from build123d import *

# Parameters (mm, degrees)
SKETCH1_R                  = 75.438
BOSS_EXTRUDE1_DEPTH        = 3.175
SKETCH2_R                  = 3.175
CUT_EXTRUDE1_DEPTH         = 107.732676875
SKETCH3_R                  = 7
SKETCH3_R_2                = 2
CUT_EXTRUDE2_DEPTH         = 107.732676875
F_1_2_0_5_DIAMETER_HOLE1_D = 12.7


with BuildPart() as part:
    # Sketch1 → Boss-Extrude1 (new body)
    with BuildSketch(Plane(origin=(0, 0, 0), x_dir=(1, 0, 0), z_dir=(0, 1, 0))):
        with Locations(Location((0, 0, 0), (0, 0, 270))):
            Circle(SKETCH1_R)
    extrude(amount=BOSS_EXTRUDE1_DEPTH)

    # Sketch2 → Cut-Extrude1 (cut, through all)
    with BuildSketch(Plane(origin=(0, 3.175, 0), x_dir=(1, 0, 0), z_dir=(0, 1, 0))):
        with Locations(Location((50.8, 0, 0), (0, 0, 270))):
            Circle(SKETCH2_R)
        with Locations(Location((-50.8, 0, 0), (0, 0, 90))):
            Circle(SKETCH2_R)
    extrude(amount=-CUT_EXTRUDE1_DEPTH, mode=Mode.SUBTRACT)

    # Sketch3 → Cut-Extrude2 (cut, through all)
    with BuildSketch(Plane(origin=(0, 3.175, 0), x_dir=(1, 0, 0), z_dir=(0, 1, 0))):
        with Locations(Location((0, 0, 0), (0, 0, 270))):
            Circle(SKETCH3_R)
        with Locations(Location((0, -11.314, 0), (0, 0, 270))):
            Circle(SKETCH3_R_2)
        with Locations(Location((-11.314, 0, 0), (0, 0, 270))):
            Circle(SKETCH3_R_2)
        with Locations(Location((11.314, 0, 0), (0, 0, 270))):
            Circle(SKETCH3_R_2)
        with Locations(Location((0, 11.314, 0), (0, 0, 270))):
            Circle(SKETCH3_R_2)
    extrude(amount=-CUT_EXTRUDE2_DEPTH, mode=Mode.SUBTRACT)

    # 1/2 (0.5) Diameter Hole1 (through all)
    with Locations(Plane(origin=(0, 3.175, 0), x_dir=(1, 0, 0), z_dir=(0, 1, 0))):
        with Locations((0, -41.73382544)):
            Hole(F_1_2_0_5_DIAMETER_HOLE1_D / 2)


solid = part.part
Design review of the part built by this model. Coordinates are the model's own, in mm. Give positions to 0.01 mm unless a question says otherwise; leave off trailing zeros. Order: outer loops, then holes, each group sorted by start corner. A loop starts at its lowest first (then second) coordinate and runs counter-clockwise, first axis right, second up. Notation, with made-up numbers: (1.5, -10.5) - (19.5, -10.5) arc R15 ccw to (19.5, 6.5) - close; hole circle Ø7 at (81, 86). An arc over 180 degrees is marked (long way). Write item = value, one per line. Start each with the question number.
Q1. We need section D-D on x = -50.8. State the section outline as (y, z) points (3 decimals).
Q2. We need section A-A on x = 0. State the section outline as (y, z) points (3 decimals).
Q3. We need section B-B on z = 0. State the section outline as (x, y) points (3 decimals).
Q4. We need section C-C on y = 2.6. State how many separate pieces and enclosed holes the cut face has, plus the area to 3 significant figures.
Q5. To check wall thickness, follow L1, parallel to X at y = 1.95, z = 0 (3 decimals); L2, parallel to X at y = 0.8, z = -4; L3, parallel to Z at x = -50.8, y = 1.45 (3 decimals). State the ranges of each line that lie inside material, in increasing order. Write a range as from..to.
Q6. Mouldability with a two-part tool opening along Z and no side actions: class faces 1 (the face through (-1.22, 1.61, -12.9)), 2 (the face through (-73.644, 1.565, -16.353)), 3 (the face through (-16, 0, -1)) as released by +Z, released by -Z, zero draft, split by the parting line, or undercut.
Working result:
q1.outline = (0, -55.77) - (3.175, -55.77) - (3.175, -3.175) - (0, -3.175) - close; (0, 3.175) - (3.175, 3.175) - (3.175, 55.77) - (0, 55.77) - close
q2.outline = (0, -75.438) - (3.175, -75.438) - (3.175, -13.314) - (0, -13.314) - close; (0, -9.314) - (3.175, -9.314) - (3.175, -7) - (0, -7) - close; (0, 7) - (3.175, 7) - (3.175, 9.314) - (0, 9.314) - close; (0, 13.314) - (3.175, 13.314) - (3.175, 35.384) - (0, 35.384) - close; (0, 48.084) - (3.175, 48.084) - (3.175, 75.438) - (0, 75.438) - close
q3.outline = (-75.438, 0) - (-53.975, 0) - (-53.975, 3.175) - (-75.438, 3.175) - close; (-47.625, 0) - (-13.314, 0) - (-13.314, 3.175) - (-47.625, 3.175) - close; (-9.314, 0) - (-7, 0) - (-7, 3.175) - (-9.314, 3.175) - close; (7, 0) - (9.314, 0) - (9.314, 3.175) - (7, 3.175) - close; (13.314, 0) - (47.625, 0) - (47.625, 3.175) - (13.314, 3.175) - close; (53.975, 0) - (75.438, 0) - (75.438, 3.175) - (53.975, 3.175) - close
q4.separate_pieces = 1
q4.enclosed_holes = 8
q4.area = 17,500 mm²
q5.L1 = -75.438..-53.975, -47.625..-13.314, -9.314..-7, 7..9.314, 13.314..47.625, 53.975..75.438
q5.L2 = -75.33..-5.74, 5.74..75.33
q5.L3 = -55.77..-3.175, 3.175..55.77
q6.face_1 = undercut
q6.face_2 = split by the parting line
q6.face_3 = zero draft
